from build123d import *

# Parameters (mm, degrees)
F0_W      = 60.96
F0_H      = 13.716
F1_DEPTH  = 16.657
F3_DEPTH  = 60.961
F5_W      = 4.5
F5_H      = 5
F4_R      = 2.25
F6_DEPTH  = 6
F7_R      = 2.25
F8_DEPTH  = 2
F9_W      = 6
F9_H      = 0.75
F10_DEPTH = 5
F11_W     = 6
F11_H     = 0.75
F12_DEPTH = 5
F13_R     = 2
F14_R     = 2
F15_DEPTH = 0.751
F16_R     = 2
F17_DEPTH = 0.751


with BuildPart() as f1:
    # F0 (on Top) → F1 (new body)
    with BuildSketch(Plane.XY):
        Rectangle(F0_W, F0_H)
    extrude(amount=F1_DEPTH)

    # F2 (on face) → F3 (cut, through all)
    with BuildSketch(Plane(origin=(-30.48, 0, 0), x_dir=(0, -1, 0), z_dir=(-1, 0, 0))):
        Polygon((-6.858, 10.657), (-0.858, 16.657), (-6.858, 16.657), align=None)
        Polygon((6.858, 16.657), (-0.5295271985, 16.657), (0.5445904681, 14.1634047031), (4.491972737, 8.7391110137), (6.858, 6.0806702822), align=None)
    extrude(amount=-F3_DEPTH, mode=Mode.SUBTRACT)

    # F5 (on face) + F4 (on face) → F6 (cut)
    with BuildSketch(Plane.XZ.offset(6.858)):
        with Locations((-27.5, 6)):
            Rectangle(F5_W, F5_H)
        with Locations((-22.5, 6)):
            Rectangle(F5_W, F5_H)
        with Locations((-17.5, 6)):
            Rectangle(F5_W, F5_H)
        with Locations((-12.5, 6)):
            Rectangle(F5_W, F5_H)
        with Locations((-7.5, 6)):
            Rectangle(F5_W, F5_H)
        with Locations((-2.5, 6)):
            Rectangle(F5_W, F5_H)
        with Locations((2.5, 6)):
            Rectangle(F5_W, F5_H)
        with Locations((7.5, 6)):
            Rectangle(F5_W, F5_H)
        with Locations((12.5, 6)):
            Rectangle(F5_W, F5_H)
        with Locations((17.5, 6)):
            Rectangle(F5_W, F5_H)
        with Locations((22.5, 6)):
            Rectangle(F5_W, F5_H)
        with Locations((27.5, 6)):
            Rectangle(F5_W, F5_H)
    with BuildSketch(Plane(origin=(0, 6.858, 0), x_dir=(-1, 0, 0), z_dir=(0, 1, 0))):
        with Locations((27.5, 5.3285)):
            Circle(F4_R)
        with Locations((22.5, 5.3285)):
            Circle(F4_R)
        with Locations((17.5, 5.3285)):
            Circle(F4_R)
        with Locations((12.5, 5.3285)):
            Circle(F4_R)
        with Locations((7.5, 5.3285)):
            Circle(F4_R)
        with Locations((2.5, 5.3285)):
            Circle(F4_R)
        with Locations((-2.5, 5.3285)):
            Circle(F4_R)
        with Locations((-7.5, 5.3285)):
            Circle(F4_R)
        with Locations((-12.5, 5.3285)):
            Circle(F4_R)
        with Locations((-17.5, 5.3285)):
            Circle(F4_R)
        with Locations((-22.5, 5.3285)):
            Circle(F4_R)
        with Locations((-27.5, 5.3285)):
            Circle(F4_R)
    extrude(amount=-F6_DEPTH, dir=(0, -1, 0), mode=Mode.SUBTRACT)

    # F7 (on face) → F8 (cut)
    with BuildSketch(Plane(origin=(0, 8.7575, 8.7575), x_dir=(1, 0, 0), z_dir=(0, 0.7071067812, 0.7071067812))):
        with Locations((-27.5, -6.9289393488)):
            Circle(F7_R)
        with Locations((-22.5, -6.9289393488)):
            Circle(F7_R)
        with Locations((-17.5, -6.9289393488)):
            Circle(F7_R)
        with Locations((-12.5, -6.9289393488)):
            Circle(F7_R)
        with Locations((-7.5, -6.9289393488)):
            Circle(F7_R)
        with Locations((-2.5, -6.9289393488)):
            Circle(F7_R)
        with Locations((2.5, -6.9289393488)):
            Circle(F7_R)
        with Locations((7.5, -6.9289393488)):
            Circle(F7_R)
        with Locations((12.5, -6.9289393488)):
            Circle(F7_R)
        with Locations((17.5, -6.9289393488)):
            Circle(F7_R)
        with Locations((22.5, -6.9289393488)):
            Circle(F7_R)
        with Locations((27.5, -6.9289393488)):
            Circle(F7_R)
    extrude(amount=-F8_DEPTH, mode=Mode.SUBTRACT)

    # F9 (on face) → F10 (join)
    with BuildSketch(Plane(origin=(-30.48, 0, 0), x_dir=(0, -1, 0), z_dir=(-1, 0, 0))):
        with Locations((0, 0.375)):
            Rectangle(F9_W, F9_H)
    extrude(amount=F10_DEPTH)

    # F11 (on face) → F12 (join)
    with BuildSketch(Plane.YZ.offset(30.48)):
        with Locations((0, 0.375)):
            Rectangle(F11_W, F11_H)
    extrude(amount=F12_DEPTH)

    # F13
    f13_edges = [f1.edges().sort_by_distance(p)[0] for p in [
        (-35.48, 3, 0.375),
        (-35.48, -3, 0.375),
        (35.48, -3, 0.375),
        (35.48, 3, 0.375),
    ]]
    fillet(f13_edges, radius=F13_R)

    # F14 (on face) → F15 (cut, through all)
    with BuildSketch(Plane.XY.offset(0.75)):
        with Locations((-33.02, 0)):
            Circle(F14_R)
    extrude(amount=-F15_DEPTH, mode=Mode.SUBTRACT)

    # F16 (on face) → F17 (cut, through all)
    with BuildSketch(Plane.XY.offset(0.75)):
        with Locations((33.02, 0)):
            Circle(F16_R)
    extrude(amount=-F17_DEPTH, mode=Mode.SUBTRACT)


solid = f1.part
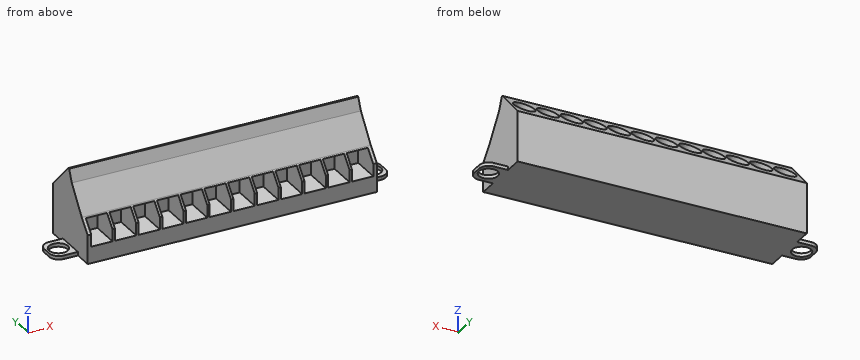
Input: part model. Units: mm. Frame: model coordinates. Give positions to 0.01 mm unless a question says otherwise; leave off trailing zeros. Order: outer loops, then holes, each group sorted by start corner. A loop starts at its lowest first (then second) coordinate and runs counter-clockwise, first axis right, second up.
Q1. Contact query for flat-ended pins moving along their axis: pin 1 Ø2.5 at (y, z) = (-3.5, 5) entering from -X; pin 2 Ø2.5 at (y, z) = (-4.5, 6.5) entering from +X; pin 3 Ø1.3 at (x, y) = (-8.5, -4.5) entering from +Z; pin 4 Ø2.5 at (x, y) = (33.02, 0) entering from -Z. Output: stop coordinate, or through.
Checked values:
pin 1: stops at x = -30.48
pin 2: stops at x = 30.48
pin 3: stops at z = 9.62
pin 4: passes through
Q2. Section B-B on x = -23. Output: boundary loops of the cut face in (y, z) (3 decimals).
Checked values:
outline: (-6.858, 0) - (6.858, 0) - (6.858, 10.657) - (5.409, 12.106) - (3.995, 10.692) - (0.893, 13.794) - (2.307, 15.208) - (0.858, 16.657) - (0.53, 16.657) - (-0.545, 14.163) - (-4.492, 8.739) - (-4.705, 8.5) - (-0.858, 8.5) - (-0.858, 3.5) - (-6.858, 3.5) - close
Q3. Ray query, probe 1 along Y at (x, z) = (33.02, 0.5); probe 2 along X at (y, z) = (0, 6.75); probe 3 along Z at (x, y) = (31, -1). Return the intervals inside material, ascending.
Checked values:
probe 1: y = -3 to -2, 2 to 3
probe 2: x = -30.48 to 30.48
probe 3: z = 0 to 0.75
Q4. Section A-A on x = 6. Output: boundary loops of the cut face in (y, z).
Checked values:
outline: (-6.86, 0) - (6.86, 0) - (6.86, 10.66) - (5.04, 12.47) - (3.63, 11.06) - (1.26, 13.43) - (2.67, 14.84) - (0.86, 16.66) - (0.53, 16.66) - (-0.54, 14.16) - (-4.49, 8.74) - (-4.7, 8.5) - (-0.86, 8.5) - (-0.86, 3.5) - (-6.86, 3.5) - close
